Geometry check sheet. Reference: the model listing, model coordinates, mm. Face numbers are marked on the shaded views. A direction names the side the tool comes from. Give positions to 0.01 mm unless a question says otherwise; leave off trailing zeros. Order: outer loops, then holes, each group sorted by start corner. A loop starts at its lowest first (then second) coordinate and runs counter-clockwise, first axis right, second up. Notation, with made-up numbers: M 22.25,43.25 L 39.25,43.25 A22 ccw 39.25,80.25 Z; hole C -15,68 d7. An arc over 180 degrees is marked long. One line per question, with ' | ' between items. Start each with the question number.
from build123d import *

# Parameters (mm, degrees)
F0_W         = 36.3061204553
F0_H         = 33.8365361094
F1_DEPTH     = 25.4
F5_DEPTH     = 50.99146
F7_T1_DEPTH  = 32.9564355705
F7_T3_DEPTH  = 33.7043488182
F7_T5_DEPTH  = 40.83146
F7_T10_DEPTH = 5.08
F7_T16_DEPTH = 5.08


# Not quite as in the source:
# - a fillet or chamfer that OpenCascade refuses, or shapes differently, is made with other operations: its cross-section is extruded or revolved along the edge and cut away or added
# - a feature of the source that left no trace in its solid (it failed there, or was rolled back) is left out


with BuildPart() as f1:
    # F0 (on Front) → F1 (new body, symmetric)
    with BuildSketch(Plane.XZ):
        with Locations((-18.1530602276, 16.9182680547)):
            Rectangle(F0_W, F0_H)
    extrude(amount=F1_DEPTH, both=True)

    # F3 (on face) → F5 (join)
    with BuildSketch(Plane(origin=(0, 25.4, 0), x_dir=(-1, 0, 0), z_dir=(0, 1, 0))):
        Polygon((36.3061204553, 33.8365361094), (17.6228713244, 52.0772151649), (0, 33.8365361094), align=None)
    extrude(amount=-F5_DEPTH)

    # F7: fillet of radius 5.08 on 5 edges, made by hand

    # F7_s2 → F7_t1 (cut)
    with BuildSketch(Plane(origin=(-30.9828597215, 0, 32.0690306362), x_dir=(0, 1, 0), z_dir=(0.6948226329, 0, -0.7191811377))):
        with BuildLine():
            ThreePointArc((-20.51146, 23.510391109), (-24.1035624484, 22.0224935574), (-25.59146, 18.430391109))
            Line((-25.59146, 18.430391109), (-25.59146, 23.510391109))
            Line((-25.59146, 23.510391109), (-20.51146, 23.510391109))
        make_face()
        with BuildLine():
            ThreePointArc((25.4, 18.430391109), (23.9121024484, 22.0224935574), (20.32, 23.510391109))
            Line((20.32, 23.510391109), (25.4, 23.510391109))
            Line((25.4, 23.510391109), (25.4, 18.430391109))
        make_face()
    extrude(amount=F7_T1_DEPTH, mode=Mode.SUBTRACT)

    # F7_s4 → F7_t3 (cut)
    with BuildSketch(Plane(origin=(-10.7619958041, 0, -10.507064916), x_dir=(0, 1, 0), z_dir=(0.7155307644, 0, 0.698581223))):
        with BuildLine():
            ThreePointArc((25.4, 44.4938565788), (23.9121024484, 48.0859590272), (20.32, 49.5738565788))
            Line((20.32, 49.5738565788), (25.4, 49.5738565788))
            Line((25.4, 49.5738565788), (25.4, 44.4938565788))
        make_face()
        with BuildLine():
            ThreePointArc((-20.51146, 49.5738565788), (-24.1035624484, 48.0859590272), (-25.59146, 44.4938565788))
            Line((-25.59146, 44.4938565788), (-25.59146, 49.5738565788))
            Line((-25.59146, 49.5738565788), (-20.51146, 49.5738565788))
        make_face()
    extrude(amount=F7_T3_DEPTH, mode=Mode.SUBTRACT)

    # F7_s6 → F7_t5 (cut)
    with BuildSketch(Plane.XZ.offset(-20.32)):
        with BuildLine():
            ThreePointArc((-14.074629897, 48.4045824879), (-17.6538784549, 49.9543417124), (-21.2768626893, 48.5097797958))
            Line((-21.2768626893, 48.5097797958), (-17.6228713244, 52.0772151649))
            Line((-17.6228713244, 52.0772151649), (-14.074629897, 48.4045824879))
        make_face()
    extrude(amount=F7_T5_DEPTH, mode=Mode.SUBTRACT)


with BuildPart() as f7_tool8:
    # F7_s9 → F7_t10 (new body)
    with BuildSketch(Plane.XZ.offset(20.51146)):
        Polygon((-17.7280700763, 44.8748835126), (-14.074629897, 48.4045824879), (-17.6228713244, 52.0772151649), (-21.2768626893, 48.5097797958), align=None)
    extrude(amount=F7_T10_DEPTH)

    # F7_s11 → F7_t12 (revolve, cut)
    with BuildSketch(Plane(origin=(-17.7280700763, -20.51146, 44.8748835126), x_dir=(-0.0146046499, 0, -0.9998933464), z_dir=(-0.9998933464, 0, 0.0146046499))):
        with BuildLine():
            ThreePointArc((0, -5.08), (5.08, 0), (0, 5.08))
            Line((0, 5.08), (0, -5.08))
        make_face()
    revolve(axis=Axis((-17.7280700763, -20.51146, 44.8748835126), (0, -1, 0)), mode=Mode.SUBTRACT)


with BuildPart() as f1_1:
    add(f1.part)

    # F7_t7: cut F7_tool8
    add(f7_tool8.part, mode=Mode.SUBTRACT)


with BuildPart() as f7_tool14:
    # F7_s15 → F7_t16 (new body)
    with BuildSketch(Plane.XZ.offset(-20.32)):
        Polygon((-17.7280700763, 44.8748835126), (-14.074629897, 48.4045824879), (-17.6228713244, 52.0772151649), (-21.2768626893, 48.5097797958), align=None)
    extrude(amount=-F7_T16_DEPTH)

    # F7_s17 → F7_t18 (revolve, cut)
    with BuildSketch(Plane(origin=(-17.7280700763, 20.32, 44.8748835126), x_dir=(-0.0146046499, 0, -0.9998933464), z_dir=(0.9998933464, 0, -0.0146046499))):
        with BuildLine():
            ThreePointArc((0, -5.08), (5.08, 0), (0, 5.08))
            Line((0, 5.08), (0, -5.08))
        make_face()
    revolve(axis=Axis((-17.7280700763, 20.32, 44.8748835126), (0, 1, 0)), mode=Mode.SUBTRACT)


with BuildPart() as f1_2:
    add(f1_1.part)

    # F7_t13: cut F7_tool14
    add(f7_tool14.part, mode=Mode.SUBTRACT)


solid = f1_2.part
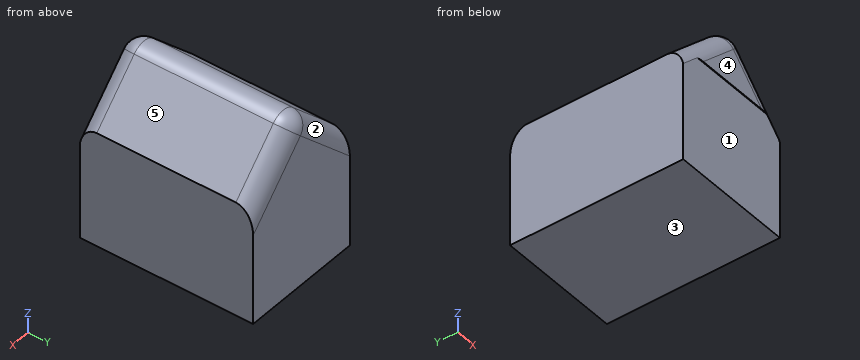
Item 1: Cross-section at A-A, the plane y = 14. Record the cut outline in (x, z), plus the area to 3 significant figures.
Item 2: Set-up check for the marked faces 1 and 2: record each of +Z, -Z, +X, -X, +Y, -Y from which the full face is reachable in a straight line by a thin tool's end or side.
Item 3: Mould release check, pull along Z, two halves, no side actions. Record for the marked faces 3, 4 and 5: released by +Z, released by -Z, zero draft, split by the parting line, or undercut.
Item 4: Depth check by flat-ended pin: pin 1 (6 mm diameter, centred on x = -7, z = 8.5, fed in from -Y). Enter the tip coordinate at first touch or a pass-through.
Item 5: Material ranges on line 1 along Y through (x, z) = (-13, 40.5); line 2 along Y through (x, z) = (-33, 21); line 3 along Z through (x, y) = (-25, 10), recorded low to high.
Outcome:
1) outline: M -36.31,0 L 0,0 L 0,33.84 L -14.07,48.4 A5.08 ccw -21.28,48.51 L -36.31,33.84 Z | area: 1,550 mm²
2) face 1: -Z, +X, -X, -Y | face 2: +Z, -X, +Y
3) face 3: released by -Z | face 4: zero draft | face 5: released by +Z
4) pin 1: stops at y = -25.4
5) line 1: y = -25.58 to 25.39 | line 2: y = -25.4 to 25.4 | line 3: z = 0 to 44.87
